Job drawing, mm, ordinate dimensions from the low corner. One solid piece. Coordinates: 2 decimals unless noted, no trailing zeros. Loops run counter-clockwise (first coordinate to the right, second up) from the corner with the lowest first, then second, coordinate; pieces in that order, holes last. Notation, with made-up numbers: M 62,-12.75 L 114,-12.75 A30 cw 114,17.25 Z; hole C -13.75,-15.5 d7. An arc over 180 degrees is marked long. Answer as a JSON object with one key per item and string values. Group by question number.
1. Mould opens along Z. For the marked faces 1 and 2 say: released by +Z, released by -Z, zero draft, split by the parting line, or undercut.
2. Saw through at B-B on x = 56. Write the cut outline in (y, z).
3. Saw through at C-C on y = 8.75. Write the cut outline in (x, z) (3 decimals).
4. Drop flat-ended pins along their axis: pin 1 Ø1 at (x, z) = (58, 55) entering from +Y; pin 2 Ø1 at (y, z) = (4.5, 44) entering from -X; pin 3 Ø18.5 at (x, z) = (20.5, 31.5) entering from +Y; pin 4 Ø12 at (x, y) = (26, 13) entering from +Z. Give the stop position or say it passes through.
5. Saw through at D-D on x = 35.5. Write the cut outline in (y, z), then the cut area to 3 significant figures.
6. Saw through at A-A on z = 34. Write the cut outline in (x, y).
7. Drill centre lines: L1, parallel to Y at x = 46.5, z = 51.5; L2, parallel to Y at x = 42, z = 3.5; L3, parallel to Z at x = 17, y = 2.5. Where is each one in solid material? Low to high.
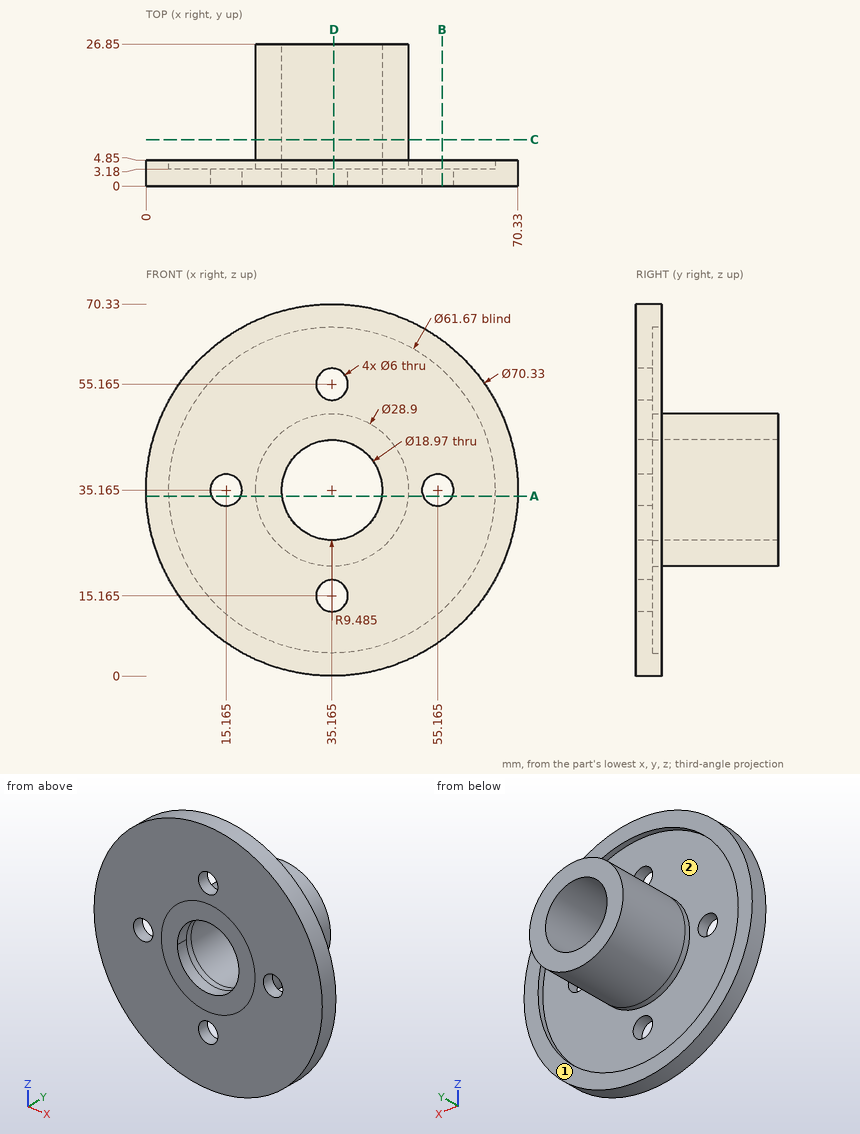
Outcome:
{
 "1": {"face 1": "zero draft", "face 2": "undercut"},
 "2": {"outline": "M 0,6.84 L 4.85,6.84 L 4.85,12.43 L 3.18,12.43 L 3.18,32.28 L 0,32.28 Z; M 0,38.05 L 3.18,38.05 L 3.18,57.9 L 4.85,57.9 L 4.85,63.49 L 0,63.49 Z"},
 "3": {"outline": "C 35.165,35.165 d28.9; hole C 35.165,35.165 d18.97"},
 "4": {"pin 1": "stops at y = 3.18", "pin 2": "stops at x = 1", "pin 3": "stops at y = 26.85", "pin 4": "stops at z = 49.26"},
 "5": {"outline": "M 0,0 L 4.85,0 L 4.85,4.33 L 3.18,4.33 L 3.18,12.18 L 0,12.18 Z; M 0,18.15 L 3.18,18.15 L 3.18,20.72 L 26.85,20.72 L 26.85,25.69 L 0,25.69 Z; M 0,44.64 L 26.85,44.64 L 26.85,49.61 L 3.18,49.61 L 3.18,52.18 L 0,52.18 Z; M 0,58.15 L 3.18,58.15 L 3.18,66 L 4.85,66 L 4.85,70.33 L 0,70.33 Z", "area": "375 mm²"},
 "6": {"outline": "M 0.02,0 L 12.4,0 L 12.4,3.18 L 4.35,3.18 L 4.35,4.85 L 0.02,4.85 Z; M 17.93,0 L 25.75,0 L 25.75,26.85 L 20.76,26.85 L 20.76,3.18 L 17.93,3.18 Z; M 44.58,0 L 52.4,0 L 52.4,3.18 L 49.57,3.18 L 49.57,26.85 L 44.58,26.85 Z; M 57.93,0 L 70.31,0 L 70.31,4.85 L 65.98,4.85 L 65.98,3.18 L 57.93,3.18 Z"},
 "7": {"L1": "y = 0 to 3.18", "L2": "y = 0 to 4.85", "L3": "z = 5.06 to 32.79, 37.54 to 65.27"}
}
